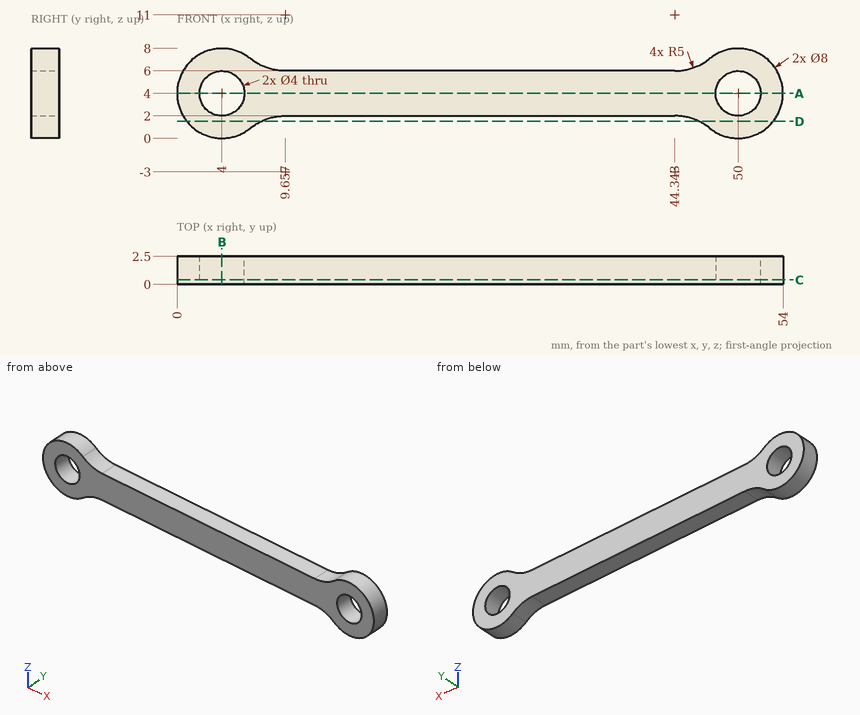
Here's the drawing with two shaded views (mm, measured from the low corner). I have some questions. Round coordinates to 2 decimals unless told otherwise and drop trailing zeros. Loops run counter-clockwise (first coordinate to the right, second up) from the corner with the lowest first, then second, coordinate; pieces in that order, holes last.
Item 1: Please list where these lines run through material, in increasing order: L1, parallel to X at y = 1.15, z = 4; L2, parallel to X at y = 2.2, z = 3.5; L3, parallel to Z at x = 19.5, y = 0.9.
Item 2: Suppose I cut it at B-B, the plane x = 4. Write out the boundary of the cut face in (y, z).
Item 3: Suppose I cut it at D-D, the plane z = 1.5. Write out the boundary of the cut face in (x, y).
Item 4: Suppose I cut it at C-C, the plane y = 0.4. Write out the boundary of the cut face in (x, z).
Item 5: Suppose I cut it at A-A, the plane z = 4. Write out the boundary of the cut face in (x, y), then the cut area to 3 significant figures.
Item 6: Will these pins go through, and if not, where does the flat tip stop? pin 1 Ø1 at (y, z) = (1, 6.5) entering from -X; pin 2 Ø1 at (x, y) = (14, 1) entering from +Z; pin 3 Ø1 at (x, y) = (46.5, 2) entering from +Z; pin 4 Ø3 at (x, z) = (50, 4) entering from +Y.
Reported:
1. L1: x = 0 to 2, 6 to 48, 52 to 54
1. L2: x = 0.03 to 2.06, 5.94 to 48.06, 51.94 to 53.97
1. L3: z = 2 to 6
2. outline: (0, 0) - (2.5, 0) - (2.5, 2) - (0, 2) - close; (0, 6) - (2.5, 6) - (2.5, 8) - (0, 8) - close
3. outline: (0.88, 0) - (7.48, 0) - (7.48, 2.5) - (0.88, 2.5) - close; (46.52, 0) - (53.12, 0) - (53.12, 2.5) - (46.52, 2.5) - close
4. outline: (6.51, 0.89) arc R5 cw to (9.66, 2) - (44.34, 2) arc R5 cw to (47.49, 0.89) arc R4 ccw (long way) to (47.49, 7.11) arc R5 cw to (44.34, 6) - (9.66, 6) arc R5 cw to (6.51, 7.11) arc R4 ccw (long way) to start; hole circle Ø4 at (4, 4); hole circle Ø4 at (50, 4)
5. outline: (0, 0) - (2, 0) - (2, 2.5) - (0, 2.5) - close; (6, 0) - (48, 0) - (48, 2.5) - (6, 2.5) - close; (52, 0) - (54, 0) - (54, 2.5) - (52, 2.5) - close
5. area: 115 mm2
6. pin 1: stops at x = 0.54
6. pin 2: stops at z = 6
6. pin 3: stops at z = 6.76
6. pin 4: passes through
